Could you check a few things on this model? Use its own coordinates, in mm. A direction names the side the tool comes from. Round coordinates to 2 decimals unless told otherwise and drop trailing zeros. Write each loop counter-clockwise with the first axis right and the second up, starting at its lowest first coordinate (ties: lowest second). Pieces come first, ordered by that corner, then holes. Notation, with made-up numbers: (-4, 42.5) - (2, 42.5) arc R8 ccw to (2, 53.5) - close; hole circle Ø11 at (-35.75, 79). An arc over 180 degrees is marked (long way). Write each question's results on one line, items separated by ' | '. Start each with the question number.
(1) On a 3-axis mill with a long thin cutter (end or side, diameter ignored), from which of +Z, -Z, +X, -X, +Y, -Y can I reach the whole of each face in a straight line? I mean faces 1 (the cylindrical face through (25.819, 19.81, -50.805)), 2 (the flat face through (6.35, 20, -79)), 3 (the flat face through (25, 25.4, -84)), 4 (the cylindrical face through (39.73, 10.25, -6.97)). Say none if no direction works.
(2) For P1, Ø7.5, axis at x = 45, z = -5, coming from the +Y side; P2, Ø3, axis at x = 6, z = -38, coming from the +Y side; P3, Ø1.4, axis at y = 19, z = -75.5, coming from the -X side; P4, Ø2.5, axis at y = 20, z = -76.5, coming from the +X side, each with a flat end and sliding along its axis, tell me the tip position at first contact or that it passes through.
(3) Please list where these lines run through material, in increasing order: line 1 (Z direction, x = 44.45, y = 4); line 2 (X direction, y = 11.75, z = -6.35); line 3 (X direction, y = 6, z = -38). Write a range as [from, to].
(4) Thinking about a two-plate mould opening in Z: for faces 5 (the cylindrical face through (22.539, 18.783, -60.765)), 6 (the cylindrical face through (1.36, 6.44, -1.43)), 7 (the flat face through (41.3, 23.8, -79.5)), which applies, +Z half, -Z half, draft (parallel to the pull), parting line (faces both ways), or undercut?
(5) Imagine slicing it at C-C on z = -34.5. Write out the boundary of the cut face in (x, y).
(6) Imagine slicing it at D-D on y = 35. Write out the boundary of the cut face in (x, z) (3 decimals).
(7) Imagine slicing it at A-A on x = 25.4. State how many separate pieces and enclosed holes the cut face has, then the cut area to 3 significant figures.
Autodesk Inventor part; units mm, degrees
ref_plane "YZ Plane" through (0, 0, 0) normal (1, 0, 0) x (0, 1, 0)
ref_plane "XZ Plane" through (0, 0, 0) normal (0, 1, 0) x (-1, 0, 0)
ref_plane "XY Plane" through (0, 0, 0) normal (0, 0, 1) x (1, 0, 0)
sketch "Sketch1" plane through (0, 0, 0) normal (0, 1, 0) x (-1, 0, 0)
  line L0 (0, 0) -> (-50.8, 0)
  line L1 (-50.8, 0) -> (-50.8, -88.9)
  line L2 (-50.8, -88.9) -> (0, -88.9)
  line L3 (0, -88.9) -> (0, 0)
  dimension "d0" = 50.8
  dimension "d1" = 88.9
extrude "Extrusion1" add sketch "Sketch1" along normal blind 12.7
sketch "Sketch2" plane through (0, 12.7, 0) normal (0, 1, 0) x (1, 0, 0)
  line L0 (50.8, 0) -> (50.8, 88.9)
  line L1 (50.8, 88.9) -> (0, 88.9)
  line L2 (0, 88.9) -> (0, 0)
  line L3 (6.35, 88.9) -> (44.45, 88.9)
  line L4 (44.45, 88.9) -> (44.45, 69.85)
  line L5 (44.45, 69.85) -> (6.35, 69.85)
  line L6 (6.35, 69.85) -> (6.35, 88.9)
  line L7 (6.35, 79.375) -> (0, 79.375) construction
  line L8 (44.45, 79.375) -> (50.8, 79.375) construction
  circle A0 centre (25.4, 69.85) radius 19.05
  dimension "d4" = 19.05
  dimension "d5" = 6.35
extrude "Extrusion2" add sketch "Sketch2" along normal blind 12.7
sketch "Sketch3" plane through (0, 25.4, 0) normal (0, 1, 0) x (1, 0, 0)
  arc A0 (6.35, 69.85) -> (44.45, 69.85) centre (25.4, 69.85) ccw
  circle A1 centre (25.4, 69.85) radius 12.7
  point P0 (0, 0)
  dimension "d8" = 25.4
extrude "Extrusion3" add sketch "Sketch3" along normal blind 12.7
sketch "Sketch6" plane through (0, 12.7, 0) normal (0, 1, 0) x (1, 0, 0)
  line L0 (0, 88.9) -> (0, 0)
  line L1 (0, 0) -> (50.8, 0)
  line L2 (50.8, 0) -> (50.8, 88.9)
  line L3 (44.45, 88.9) -> (44.45, 6.35) construction
  line L4 (44.45, 6.35) -> (6.35, 6.35) construction
  line L5 (6.35, 6.35) -> (6.35, 88.9) construction
  line L6 (6.35, 38.1) -> (44.45, 38.1) construction
  dimension "d35" = 6.35
  dimension "d36" = 31.75
hole "Hole3" at (25.4, 38.1, -69.85) direction (0, -1, 0) diameter 19.05 end through all
sketch "Sketch7" plane through (50.8, 0, -88.9) normal (0, 0, -1) x (-1, 0, 0)
  line L0 (0, 0) -> (0, 12.7)
  line L1 (44.45, 12.7) -> (6.35, 12.7) construction
  point P0 (25.4, 12.7)
hole "Hole4" at (25.4, 12.7, -88.9) direction (0, 0, 1) diameter 4.9784 end up to surface
hole "Hole5" at (6.35, 12.7, -6.35) at (6.35, 12.7, -38.1) at (44.45, 12.7, -6.35) at (44.45, 12.7, -38.1) direction (0, -1, 0) diameter 5.1054 end through all counterbore diameter 9.525 counterbore depth 4.826
fillet "Fillet1" radius 4.7625 5 edges at (25.4, 12.7, -50.8) (6.35, 12.7, -79.375) (44.45, 12.7, -79.375) (0, 6.35, 0) (50.8, 6.35, 0)
chamfer "Chamfer1" distance 6.35 distance2 3.175 3 edges at (44.45, 25.4, -79.375) (25.4, 25.4, -50.8) (6.35, 25.4, -79.375) measured on face at (24.8897, 25.4, -86.7525)
properties part number "Fillet Chamfer Complete"
Response:
1) face 1: +Z, +Y | face 2: +Z, -Z, -X, +Y | face 3: -Z, +Y | face 4: +Y
2) P1: y = 12.7 | P2: through | P3: x = 6.35 | P4: x = 44.45
3) line 1: [-88.9, -40.65], [-35.55, -8.9], [-3.8, 0] | line 2: [0, 1.59], [11.11, 39.69], [49.21, 50.8] | line 3: [0, 3.8], [8.9, 41.9], [47, 50.8]
4) face 5: undercut | face 6: +Z half | face 7: draft
5) outline: (0, 0) - (50.8, 0) - (50.8, 12.7) - (47.57, 12.7) - (47.57, 7.87) - (41.33, 7.87) - (41.33, 12.7) - (9.47, 12.7) - (9.47, 7.87) - (3.23, 7.87) - (3.23, 12.7) - (0, 12.7) - close
6) outline: circle Ø25.4 at (25.4, -69.85); hole circle Ø19.05 at (25.4, -69.85)
7) separate pieces: 3 | enclosed holes: 0 | area: 1,160 mm²
